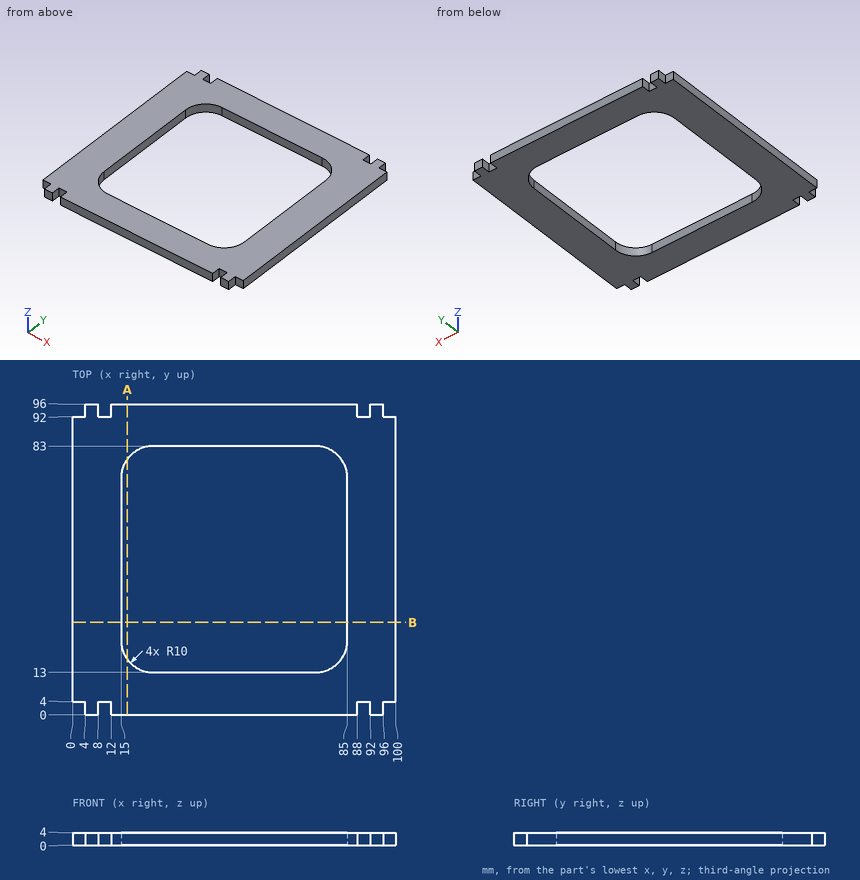
Source: three-view drawing plus pictorial views. Frame: mm from the lowest corner of the part. Round coordinates to 2 decimals unless told otherwise and drop trailing zeros. Order: outer loops, then holes, each group sorted by start corner. A loop starts at its lowest first (then second) coordinate and runs counter-clockwise, first axis right, second up. Notation, with made-up numbers: (-22, 43.5) - (-18, 43.5) arc R21 ccw to (-18, 54.5) - close; hole circle Ø9 at (86, 55.25). An arc over 180 degrees is marked (long way). Answer in a Markdown table with one row per item.
Item 1: Section query A-A (x = 17). Return the cut outline in (y, z).
Model answer:
| item | result |
|---|---|
| outline | (0, 0) - (17, 0) - (17, 4) - (0, 4) - close; (79, 0) - (96, 0) - (96, 4) - (79, 4) - close |
Item 2: Pin query (flat end, axial travel): pin 1 (1.2 mm diameter, centred on x = 11, z = 2, fed in from -Y); pin 2 (1.2 mm diameter, centred on x = 49, z = 2.5, fed in from -Y); pin 3 (2 mm diameter, centred on x = 90.5, z = 2.5, fed in from +Y); pin 4 (1.2 mm diameter, centred on y = 2, z = 1, fed in from -X). Return the tip coordinate at first contact, or that it passes through.
Model answer:
| item | result |
|---|---|
| pin 1 | stops at y = 4 |
| pin 2 | stops at y = 0 |
| pin 3 | stops at y = 92 |
| pin 4 | stops at x = 4 |
Item 3: Section query B-B (y = 28.5). Return the cut outline in (x, z).
Model answer:
| item | result |
|---|---|
| outline | (0, 0) - (15, 0) - (15, 4) - (0, 4) - close; (85, 0) - (100, 0) - (100, 4) - (85, 4) - close |
Item 4: Line query: line 1 (Y direction, x = 57, z = 1.3); line 2 (X direction, y = 31.5, z = 0.7); line 3 (X direction, y = 75.5, z = 2.1). Output: solid intervals per line, ascending.
Model answer:
| item | result |
|---|---|
| line 1 | y = 0 to 13, 83 to 96 |
| line 2 | x = 0 to 15, 85 to 100 |
| line 3 | x = 0 to 15.32, 84.68 to 100 |
